```python
from build123d import *

# Parameters (mm, degrees)
F1_DEPTH = 19
F2_DEPTH = 2
F3_DEPTH = 0.6


with BuildPart() as f1:
    # F0 (on Top) → F1 (new body)
    with BuildSketch(Plane.XY):
        Polygon((920.027071, -297.317977), (920.027071, -295.269437), (-49.972929, -510.269437), (-49.972929, -512.317977), align=None)
        Polygon((-49.972929, 510.269437), (920.027071, 295.269437), (920.027071, 297.317977), (-49.972929, 512.317977), align=None)
    extrude(amount=-F1_DEPTH)

    # F0 (on Top) → F2 (join)
    with BuildSketch(Plane.XY):
        Polygon((-49.972929, 512.317977), (920.027071, 297.317977), (920.027071, 305), (920.027071, 314.730563), (-49.972929, 529.730563), (-49.972929, 520), align=None)
        Polygon((920.027071, -305), (920.027071, -297.317977), (-49.972929, -512.317977), (-49.972929, -520), (-49.972929, -529.730563), (920.027071, -314.730563), align=None)
    extrude(amount=-F2_DEPTH)

    # F0 (on Top) → F3 (join)
    with BuildSketch(Plane.XY):
        Polygon((920.027071, -295.269437), (920.027071, 0), (920.027071, 295.269437), (-49.972929, 510.269437), (-49.972929, 0), (-49.972929, -510.269437), align=None)
        Polygon((920.027071, -297.317977), (920.027071, -295.269437), (-49.972929, -510.269437), (-49.972929, -512.317977), align=None)
        Polygon((920.027071, -305), (920.027071, -297.317977), (-49.972929, -512.317977), (-49.972929, -520), (-49.972929, -529.730563), (920.027071, -314.730563), align=None)
        Polygon((-49.972929, 510.269437), (920.027071, 295.269437), (920.027071, 297.317977), (-49.972929, 512.317977), align=None)
        Polygon((-49.972929, 512.317977), (920.027071, 297.317977), (920.027071, 305), (920.027071, 314.730563), (-49.972929, 529.730563), (-49.972929, 520), align=None)
    extrude(amount=F3_DEPTH)


solid = f1.part
```
Design review of the part built by this model. Coordinates are the model's own, in mm. A direction names the side the tool comes from. Coordinates: 2 decimals unless noted, no trailing zeros. Order: outer loops, then holes, each group sorted by start corner. A loop starts at its lowest first (then second) coordinate and runs counter-clockwise, first axis right, second up.
1) Take a section at A-A, the plane z = -15.75. Give the boundary of the cut face in (x, y).
2) Wall thickness on line 1 along Z through (x, y) = (12.5, 75); line 2 along Y through (x, z) = (184.5, -16.25); line 3 along Y through (x, z) = (242.5, -14.75): over which ranges is each line inside the solid? List them lowest first.
3) Take a section at B-B, the plane x = 538. Give the boundary of the cut face in (y, z), and give its area (3 significant figures).
4) Clearance check with flat-ended pins moving along their axes: pin 1 (8 mm diameter, centred on x = 121, y = 275, fed in from -Z); pin 2 (2 mm diameter, centred on x = 734, z = -9, fed in from +Y); pin 3 (4 mm diameter, centred on x = 395, z = -5.5, fed in from +Y); pin 4 (4 mm diameter, centred on y = -28, z = -3, fed in from -X). State where each tip first meets the part, or that it passes through.
5) Mouldability with a two-part tool opening along Y and no side actions: class faces 1 (the flat face through (441.817, 420.726, -0.718)), 2 (the flat face through (428, 7, 0.6)), 3 (the flat face through (441.817, -401.264, -9.367)) as +Y half, -Y half, draft (parallel to the pull), parting line (faces both ways), or undercut.
6) For faces 4 (the flat face through (433, 414, -2)), 5 (the flat face through (428.237, 404.274, -9.367)), 6 (the flat face through (428.237, -423.736, -0.718)), 7 (the flat face through (433, 404, -19)), 8 (the flat face through (433, -413, -2)), list the 3-axis set-ups (+Z, -Z, +X, -X, +Y, -Y) from which the entire face can be reached by the end or side of a thin tool; tool diameter is ignored.
7) Take a section at C-C, the plane y = 202. Give the boundary of the cut face in (x, z).
8) Take a section at D-D, the plane x = 380. Give the boundary of the cut face in (y, z), and give its area (3 significant figures).
Returned:
1. outline: (-49.97, -512.32) - (920.03, -297.32) - (920.03, -295.27) - (-49.97, -510.27) - close; (-49.97, 510.27) - (920.03, 295.27) - (920.03, 297.32) - (-49.97, 512.32) - close
2. line 1: z = 0 to 0.6
2. line 2: y = -460.35 to -458.3, 458.3 to 460.35
2. line 3: y = -447.49 to -445.44, 445.44 to 447.49
3. outline: (-399.41, -2) - (-381.99, -2) - (-381.99, -19) - (-379.95, -19) - (-379.95, 0) - (379.95, 0) - (379.95, -19) - (381.99, -19) - (381.99, -2) - (399.41, -2) - (399.41, 0.6) - (-399.41, 0.6) - close
3. area: 627 mm2
4. pin 1: stops at z = 0
4. pin 2: stops at y = 338.77
4. pin 3: stops at y = 414.13
4. pin 4: passes through
5. face 1: +Y half
5. face 2: draft
5. face 3: undercut
6. face 4: -Z, +X, +Y
6. face 5: -Z, -X
6. face 6: +Z, -Z, +X, -Y
6. face 7: -Z, +X, -X, +Y, -Y
6. face 8: -Z, +X, -Y
7. outline: (-49.97, 0) - (920.03, 0) - (920.03, 0.6) - (-49.97, 0.6) - close
8. outline: (-434.43, -2) - (-417.01, -2) - (-417.01, -19) - (-414.97, -19) - (-414.97, 0) - (414.97, 0) - (414.97, -19) - (417.01, -19) - (417.01, -2) - (434.43, -2) - (434.43, 0.6) - (-434.43, 0.6) - close
8. area: 669 mm2
